Verification items for the finished model (mm, model axes). Face numbers are marked on the shaded views. A direction names the side the tool comes from. Give positions to 0.01 mm unless a question says otherwise; leave off trailing zeros. Order: outer loops, then holes, each group sorted by start corner. A loop starts at its lowest first (then second) coordinate and runs counter-clockwise, first axis right, second up. Notation, with made-up numbers: (57, 15) -> (76, 15) arc R27 cw to (76, 37) -> close; hole circle Ø2 at (69, 42.25). An arc over 180 degrees is marked (long way). One line per question, with ' | ' between items. Start each with the question number.
Q1. Go/stop test with flat-tipped pins: pin 1 (2.5 mm diameter, centred on x = 0, y = 47.5, fed in from +Z); pin 2 (1.5 mm diameter, centred on x = -17, z = 3, fed in from -Y); pin 3 (4 mm diameter, centred on x = 12, y = 28, fed in from -Z); pin 4 (1.5 mm diameter, centred on y = 6.5, z = 2, fed in from +X). Record where each tip stops, or that it passes through.
Q2. Section check D-D on y = 27.5. Record the cut outline in (x, z).
Q3. Mould release check, pull along Y, two halves, no side actions. Record for the marked faces 1, 2, 3 and 4: released by +Y, released by -Y, zero draft, split by the parting line, or undercut.
Q4. Access from +Z, -Z, +X, -X, +Y, -Y to the whole of each face (thin tool, end or side, straight path). Record for the marked faces 5, 6 and 7.
Q5. Section check C-C on z = 3.75. Give the number of separate pieces and of enclosed holes in the cut face, plus the area to 3 significant figures.
Q6. Section check A-A on y = 7.5. Record the cut outline in (x, z).
Q7. Section check B-B on x = 0. Record the cut outline in (y, z).
Q8. Material ranges on probe 1 along Y at (x, z) = (0, 3.05); probe 2 along X at (y, z) = (24.5, 0.55); probe 3 along X at (y, z) = (48, 2.5), recorded low to high. Write a range as [from, to].
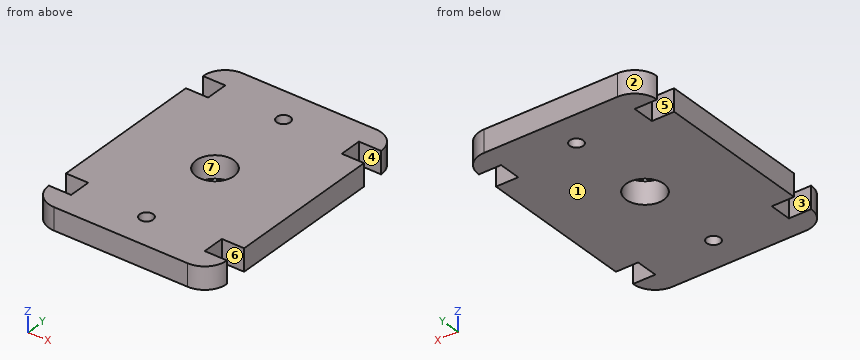
from build123d import *

# Parameters (mm, degrees)
ESQUISSE1_R        = 1.5
ESQUISSE1_R_2      = 4.25
BOSS_EXTRU_1_DEPTH = 5
CONG_1_R           = 5


with BuildPart() as part:
    # Esquisse1 → Boss.-Extru.1 (new body)
    with BuildSketch(Plane.XY):
        Polygon((-20, 0), (20, 0), (20, 5), (15, 5), (15, 10), (20, 10), (20, 45), (15, 45), (15, 50), (20, 50), (20, 55), (-20, 55), (-20, 50), (-15, 50), (-15, 45), (-20, 45), (-20, 10), (-15, 10), (-15, 5), (-20, 5), align=None)
        with Locations((0, 47.5)):
            Circle(ESQUISSE1_R, mode=Mode.SUBTRACT)
        with Locations((0, 7.5)):
            Circle(ESQUISSE1_R, mode=Mode.SUBTRACT)
        with Locations((0, 27.5)):
            Circle(ESQUISSE1_R_2, mode=Mode.SUBTRACT)
    extrude(amount=BOSS_EXTRU_1_DEPTH)

    # Congé1
    cong_1_edges = [part.edges().sort_by_distance(p)[0] for p in [
        (20, 55, 2.5),
        (20, 0, 2.5),
        (-20, 0, 2.5),
        (-20, 55, 2.5),
    ]]
    fillet(cong_1_edges, radius=CONG_1_R - 0.0001)  # a hair under: the kernel refuses the full size


solid = part.part
Filled in:
1) pin 1: through | pin 2: y = 0.16 | pin 3: z = 0 | pin 4: x = 15
2) outline: (-20, 0) -> (-4.25, 0) -> (-4.25, 5) -> (-20, 5) -> close; (4.25, 0) -> (20, 0) -> (20, 5) -> (4.25, 5) -> close
3) face 1: zero draft | face 2: released by +Y | face 3: undercut | face 4: undercut
4) face 5: +Z, -Z, -X | face 6: +Z, -Z, +X | face 7: +Z, -Z
5) separate pieces: 1 | enclosed holes: 3 | area: 2,010 mm²
6) outline: (-15, 0) -> (-1.5, 0) -> (-1.5, 5) -> (-15, 5) -> close; (1.5, 0) -> (15, 0) -> (15, 5) -> (1.5, 5) -> close
7) outline: (0, 0) -> (6, 0) -> (6, 5) -> (0, 5) -> close; (9, 0) -> (23.25, 0) -> (23.25, 5) -> (9, 5) -> close; (31.75, 0) -> (46, 0) -> (46, 5) -> (31.75, 5) -> close; (49, 0) -> (55, 0) -> (55, 5) -> (49, 5) -> close
8) probe 1: [0, 6], [9, 23.25], [31.75, 46], [49, 55] | probe 2: [-20, -3.01], [3.01, 20] | probe 3: [-15, -1.41], [1.41, 15]
